Can you work these out from the model? Positions are in its coordinate system, mm. Round coordinates to 2 decimals unless told otherwise and drop trailing zeros. Answer in a Markdown table with one row per item. Add a question column.
(1) I'm going to push flat-ended pins straight in: pin 1 (10 mm diameter, centred on x = 12.5, z = 8, fed in from -Y); pin 2 (1 mm diameter, centred on x = -7, z = 24.5, fed in from -Y); pin 3 (4 mm diameter, centred on x = -28.5, z = 12, fed in from +Y). Where does each tip first touch, or does it pass through?
(2) If we mould it in two halves opening along X, with no side actions, what happens to faces 1 (the face through (-46, -3, 50.8)), 2 (the face through (0, 1, 2.54))? For each: released by +X, released by -X, zero draft, split by the parting line, or undercut.
(3) If I drill on probe 1 along Z at (x, y) = (-16, -7.5); probe 2 along X at (y, z) = (-9.5, 11); probe 3 along X at (y, z) = (15.5, 16.5), over which ranges is the centre line in solid material (lowest first)?
from build123d import *

# Parameters (mm, degrees)
F0_W = 50.8
F0_H = 59.9056573934
F4_T = 2.54


# Not quite as in the source:
# - the arcs of a loft's sections are written as splines that run evenly, so that the points pair up as in the source's solid
# - a shell that OpenCascade refuses in one call is made with other operations: the cavity is built on its own and cut out


with BuildPart() as f3:
    # F2 (on offset) → F3 section 0
    with BuildSketch(Plane.XY.offset(50.8)):
        with BuildLine():
            add(Edge.make_bspline(
                [(31.3033898449, 36.9143729784), (28.8873497832, 38.9631750527), (26.269585061, 40.7739731742), (20.7309490894, 43.8501509409), (17.8102147937, 45.1154545216), (11.7778696482, 47.0519901199), (8.66640796, 47.7231742528), (2.3721732815, 48.4456477056), (-0.8104440715, 48.4969191609), (-7.1246843741, 47.9775662186), (-10.2561511918, 47.406954663), (-16.3477444048, 45.6657337679), (-19.3077201735, 44.4951674836), (-24.9425697859, 41.5989927782), (-27.6173042968, 39.8734559709), (-32.5788661981, 35.9336258251), (-34.865570904, 33.7194299066), (-36.9143729784, 31.3033898449)],
                knots=[0, 0, 0, 0, 0.125, 0.125, 0.25, 0.25, 0.375, 0.375, 0.5, 0.5, 0.625, 0.625, 0.75, 0.75, 0.875, 0.875, 1, 1, 1, 1], degree=3))
            add(Edge.make_bspline(
                [(-36.9143729784, 31.3033898449), (-38.9631750527, 28.8873497832), (-40.7739731742, 26.269585061), (-43.8501509409, 20.7309490894), (-45.1154545216, 17.8102147937), (-47.0519901199, 11.7778696482), (-47.7231742528, 8.66640796), (-48.4456477056, 2.3721732815), (-48.4969191609, -0.8104440715), (-47.9775662186, -7.1246843741), (-47.406954663, -10.2561511918), (-45.6657337679, -16.3477444048), (-44.4951674836, -19.3077201735), (-41.5989927782, -24.9425697859), (-39.8734559709, -27.6173042968), (-35.9336258251, -32.5788661981), (-33.7194299066, -34.865570904), (-31.3033898449, -36.9143729784)],
                knots=[0, 0, 0, 0, 0.125, 0.125, 0.25, 0.25, 0.375, 0.375, 0.5, 0.5, 0.625, 0.625, 0.75, 0.75, 0.875, 0.875, 1, 1, 1, 1], degree=3))
            add(Edge.make_bspline(
                [(-31.3033898449, -36.9143729784), (-28.8873497832, -38.9631750527), (-26.269585061, -40.7739731742), (-20.7309490894, -43.8501509409), (-17.8102147937, -45.1154545216), (-11.7778696482, -47.0519901199), (-8.66640796, -47.7231742528), (-2.3721732815, -48.4456477056), (0.8104440715, -48.4969191609), (7.1246843741, -47.9775662186), (10.2561511918, -47.406954663), (16.3477444048, -45.6657337679), (19.3077201735, -44.4951674836), (24.9425697859, -41.5989927782), (27.6173042968, -39.8734559709), (32.5788661981, -35.9336258251), (34.865570904, -33.7194299066), (36.9143729784, -31.3033898449)],
                knots=[0, 0, 0, 0, 0.125, 0.125, 0.25, 0.25, 0.375, 0.375, 0.5, 0.5, 0.625, 0.625, 0.75, 0.75, 0.875, 0.875, 1, 1, 1, 1], degree=3))
            add(Edge.make_bspline(
                [(36.9143729784, -31.3033898449), (38.9631750527, -28.8873497832), (40.7739731742, -26.269585061), (43.8501509409, -20.7309490894), (45.1154545216, -17.8102147937), (47.0519901199, -11.7778696482), (47.7231742528, -8.66640796), (48.4456477056, -2.3721732815), (48.4969191609, 0.8104440715), (47.9775662186, 7.1246843741), (47.406954663, 10.2561511918), (45.6657337679, 16.3477444048), (44.4951674836, 19.3077201735), (41.5989927782, 24.9425697859), (39.8734559709, 27.6173042968), (35.9336258251, 32.5788661981), (33.7194299066, 34.865570904), (31.3033898449, 36.9143729784)],
                knots=[0, 0, 0, 0, 0.125, 0.125, 0.25, 0.25, 0.375, 0.375, 0.5, 0.5, 0.625, 0.625, 0.75, 0.75, 0.875, 0.875, 1, 1, 1, 1], degree=3))
        make_face()
    # F0 (on Top) → F3 section 1
    with BuildSketch(Plane.XY):
        Rectangle(F0_W, F0_H)
    loft(ruled=True)

    # F4: shell of thickness 2.54, made by hand


with BuildPart() as f4_core1:
    # F4_t2: copy of F3
    add(f3.part)

    # the walls: a layer under each face that stays
    f4_faces = [f4_core1.faces().sort_by_distance(p)[0] for p in [
        (-1.9837821114, 39.0950356932, 25.4),
        (-36.8186213449, -1.9837821114, 25.4),
        (1.9837821114, -39.0950356932, 25.4),
        (36.8186213449, 1.9837821114, 25.4),
        (0, 0, 0),
    ]]
    thicken(f4_faces, amount=-F4_T, mode=Mode.SUBTRACT)


with BuildPart() as f3_1:
    add(f3.part)

    # what is left inside the walls is the cavity
    f4_cavity = [f4_core1.part.solids().sort_by_distance(p)[0] for p in [
        (11.647477, -9.877061, 50.7746),
    ]]
    add(f4_cavity, mode=Mode.SUBTRACT)


solid = f3_1.part
Calculated:
| question | item | result |
|---|---|---|
| 1 | pin 1 | y = -33.81 |
| 1 | pin 2 | y = -38.8 |
| 1 | pin 3 | y = 30.75 |
| 2 | face 1 | zero draft |
| 2 | face 2 | undercut |
| 3 | probe 1 | 0 to 2.54 |
| 3 | probe 2 | -29.92 to -27.16, 27.45 to 30.22 |
| 3 | probe 3 | -32.05 to -29.29, 28.69 to 31.44 |
